Autodesk Inventor part; units mm, degrees
ref_plane "YZ Plane" through (0, 0, 0) normal (1, 0, 0) x (0, 1, 0)
ref_plane "XZ Plane" through (0, 0, 0) normal (0, 1, 0) x (-1, 0, 0)
ref_plane "XY Plane" through (0, 0, 0) normal (0, 0, 1) x (1, 0, 0)
sketch "Sketch1" plane through (0, 0, 0) normal (0, 0, 1) x (1, 0, 0)
  line L0 (-9, 0) -> (-9, 0)
  line L1 (-18, 9) -> (-18, 69)
  line L2 (-9, 78) -> (-9, 78)
  line L3 (0, 69) -> (0, 9)
  circle A0 centre (-9, 38) radius 4
  arc A1 (-18, 9) -> (-9, 0) centre (-9, 9) ccw
  arc A2 (-9, 0) -> (0, 9) centre (-9, 9) ccw
  arc A3 (0, 69) -> (-9, 78) centre (-9, 69) ccw
  arc A4 (-9, 78) -> (-18, 69) centre (-9, 69) ccw
  circle A5 centre (-9, 9) radius 4
  circle A6 centre (-9, 69) radius 4
  point P0 (0, 0)
  point P1 (-18, 78)
  point P2 (-18, 0)
  point P3 (0, 78)
  dimension "d0" = 18
  dimension "d1" = 78
  dimension "d2" = 8
  dimension "d3" = 9
  dimension "d4" = 8
  dimension "d5" = 8
extrude "Extrusion1" add sketch "Sketch1" along normal blind 4
properties part number "zawieszenie ramie 2"
Geometry: final body of the model. Coordinates: model frame, mm. Give positions to 0.01 mm unless a question says otherwise; leave off trailing zeros. Loops run counter-clockwise (first coordinate to the right, second up) from the corner with the lowest first, then second, coordinate; pieces in that order, holes last. Notation, with made-up numbers: M -7,53.5 L 19,53.5 A18 cw 19,81.5 Z; hole C 52,65 d4. An arc over 180 degrees is marked long. Put each result on its own line as item: value.
1) Material intervals for L1, parallel to Y at x = -9, z = 1.3; L2, parallel to Y at x = -9.75, z = 0.3; L3, parallel to X at y = 39.5, z = 2.15, sorted ascending. Write a range as from..to.
Computed values:
L1: y = 0..5, 13..34, 42..65, 73..78
L2: y = 0.03..5.07, 12.93..34.07, 41.93..65.07, 72.93..77.97
L3: x = -18..-12.71, -5.29..0
2) Cut plane A-A, the plane x = -9. Return the cut outline in (y, z), plus the area to 3 significant figures.
Computed values:
outline: M 0,0 L 5,0 L 5,4 L 0,4 Z; M 13,0 L 34,0 L 34,4 L 13,4 Z; M 42,0 L 65,0 L 65,4 L 42,4 Z; M 73,0 L 78,0 L 78,4 L 73,4 Z
area: 216 mm^2
3) First-contact query: P1, Ø3, axis at x = -14.5, y = 62, coming from the -Z side; P2, Ø1.5, axis at x = -3.5, z = 1, coming from the +Y side. Flat tips, straight axial feed; report the tip coordinate or a pass-through.
Computed values:
P1: stops at z = 0
P2: stops at y = 76.64
4) Cut plane C-C, the plane z = 2.15. Return the cut outline in (x, y).
Computed values:
outline: M -18,9 A9 ccw 0,9 L 0,69 A9 ccw -18,69 Z; hole C -9,9 d8; hole C -9,38 d8; hole C -9,69 d8
5) Cut plane B-B, the plane y = 38. Return the cut outline in (x, z), plus the area to 3 significant figures.
Computed values:
outline: M -18,0 L -13,0 L -13,4 L -18,4 Z; M -5,0 L 0,0 L 0,4 L -5,4 Z
area: 40.0 mm^2
6) Mould query, pull axis X, two halves, no side actions, for faces 1 (the cylindrical face through (-12.2, 11.4, 2)), 2 (the flat face through (0, 39, 2)), 3 (the cylindrical face through (-9, 0, 2)). Classes: released by +X, released by -X, zero draft, split by the parting line, or undercut.
Computed values:
face 1: undercut
face 2: released by +X
face 3: split by the parting line
